Study the drawing (mm; zero at the part's minimum x, y, z) and answer. Round coordinates to 2 decimals unless told otherwise and drop trailing zeros. Write each loop counter-clockwise with the first axis right and the second up, starting at its lowest first coordinate (ties: lowest second). Pieces come first, ordered by that corner, then holes.
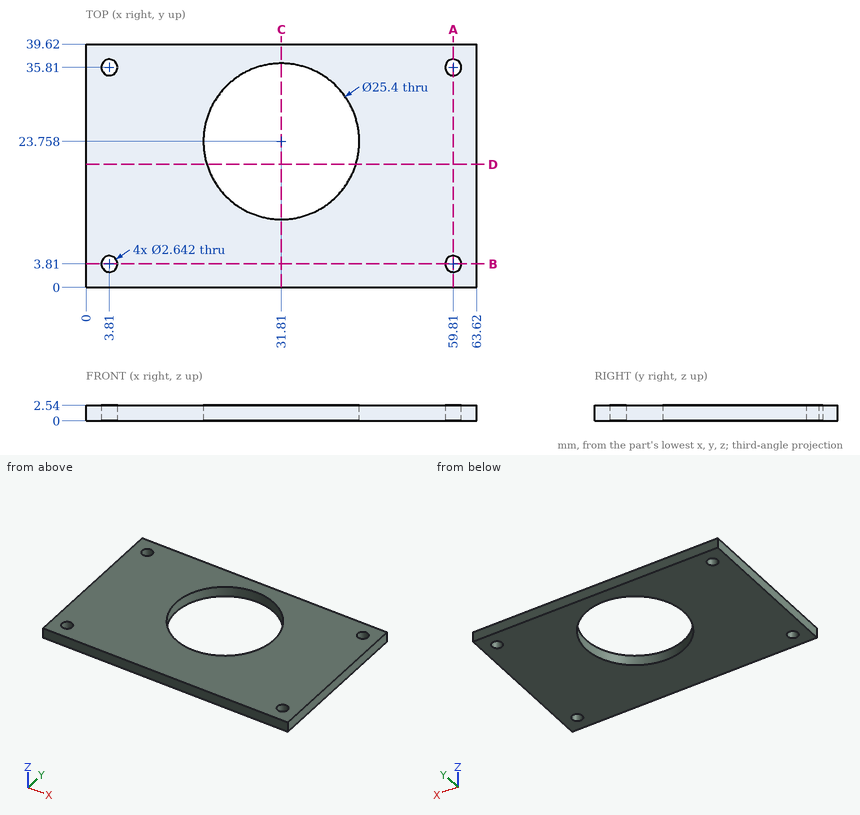
1. Section B-B on y = 3.81 is taken. Determine the outline of the cut face in (x, z).
Geometry says:
outline: (0, 0) - (2.49, 0) - (2.49, 2.54) - (0, 2.54) - close; (5.13, 0) - (58.49, 0) - (58.49, 2.54) - (5.13, 2.54) - close; (61.13, 0) - (63.62, 0) - (63.62, 2.54) - (61.13, 2.54) - close
2. Section A-A on x = 59.81 is taken. Determine the outline of the cut face in (y, z).
Geometry says:
outline: (0, 0) - (2.49, 0) - (2.49, 2.54) - (0, 2.54) - close; (5.13, 0) - (34.49, 0) - (34.49, 2.54) - (5.13, 2.54) - close; (37.13, 0) - (39.62, 0) - (39.62, 2.54) - (37.13, 2.54) - close
3. Section C-C on x = 31.81 is taken. Determine the outline of the cut face in (y, z), plus the area to 3 significant figures.
Geometry says:
outline: (0, 0) - (11.06, 0) - (11.06, 2.54) - (0, 2.54) - close; (36.46, 0) - (39.62, 0) - (39.62, 2.54) - (36.46, 2.54) - close
area: 36.1 mm2
4. Section D-D on y = 20 is taken. Determine the outline of the cut face in (x, z).
Geometry says:
outline: (0, 0) - (19.68, 0) - (19.68, 2.54) - (0, 2.54) - close; (43.94, 0) - (63.62, 0) - (63.62, 2.54) - (43.94, 2.54) - close
5. Straight lines are drawn through the part: line 1 along X through (y, z) = (3.81, 1.4); line 2 along Y through (x, z) = (60, 1.6); line 3 along X through (y, z) = (24, 1.95). For each, find the intervals that lie inside material, in ascending order.
Geometry says:
line 1: x = 0 to 2.49, 5.13 to 58.49, 61.13 to 63.62
line 2: y = 0 to 2.5, 5.12 to 34.5, 37.12 to 39.62
line 3: x = 0 to 19.11, 44.51 to 63.62
